Geometry: final body of the model. Coordinates: model frame, mm. A direction names the side the tool comes from. Give positions to 0.01 mm unless a question says otherwise; leave off trailing zeros. Write each loop counter-clockwise with the first axis right and the second up, starting at its lowest first coordinate (ties: lowest second). Pieces come first, ordered by that corner, then holes. Notation, with made-up numbers: M 30.25,52 L 49.25,52 A26 cw 49.25,82 Z; hole C 21,50.5 d7. An arc over 180 degrees is marked long. Use a Markdown table: item, result. Add a question column.
1) Set-up query: faces 4 (the flat face through (-103, 56, 20)), 5 (the flat face through (-201.182, 5.708, 8.948)), 6 (the flat face through (-82.379, 80.196, 19.088)), 7 (the cylindrical face through (-11.492, 18.486, 9.251)). Return all of +Z, -Z, +X, -X, +Y, -Y with unobstructed straight access to the full face (end or side cutting, diameter ignored); none if empty.
2) Section A-A on x = -62. Return the cut outline in (y, z), then the cut area to 3 significant figures.
3) Line query: line 1 (X direction, y = 16.5, z = 17); line 2 (Y direction, x = -67, z = 13). Output: solid intervals per line, ascending.
4) Pin query (flat end, axial travel): pin 1 (1.3 mm diameter, centred on x = -12.5, y = 16.5, fed in from -Z); pin 2 (5 mm diameter, centred on y = 73.5, z = 6.5, fed in from +X). Return the tip coordinate at first contact, or that it passes through.
5) Section D-D on y = 7. Return the cut outline in (x, z) (3 decimals).
6) Draft query along Y for faces 1 (the flat face through (-101, 1.85, 9)), 2 (the flat face through (-107, 96, 0)), 3 (the flat face through (-7.45, 95.64, 12.18)). Return one class per face: +Y half, -Y half, draft (parallel to the pull), parting line (faces both ways), or undercut.
7) Section B-B on y = 65. Return the cut outline in (x, z).
8) Section C-C on z = 9. Return the cut outline in (x, y), then the cut area to 3 significant figures.
```python
from build123d import *

# Parameters (mm, degrees)
PAD_DEPTH       = 20
POCKET_DEPTH    = 20
POCKET001_DEPTH = 18.15
SKETCH003_R     = 2.25
PAD001_DEPTH    = 18.05


with BuildPart() as part:
    # Sketch → Pad (new body)
    with BuildSketch(Plane.XY):
        Polygon((-8.910891, 97.1), (0, 88.189109), (0, 8.910891), (-8.910891, 0), (-198.089109, 0), (-207, 8.910891), (-207, 88.189109), (-198.089109, 97.1), align=None)
    extrude(amount=PAD_DEPTH)

    # Sketch001 (on Face10 of Pad) → Pocket (cut)
    with BuildSketch(Plane.XY.offset(20)):
        Polygon((-95.65, 66.925), (-95.65, 30.175), (-69.475, 4), (-33.025, 4), (-6.85, 30.175), (-6.85, 66.925), (-33.025, 93.1), (-69.475, 93.1), align=None)
        Polygon((-197.45, 66.925), (-197.45, 30.175), (-171.275, 4), (-134.825, 4), (-108.65, 30.175), (-108.65, 66.925), (-134.825, 93.1), (-171.275, 93.1), align=None)
    extrude(amount=-POCKET_DEPTH, mode=Mode.SUBTRACT)

    # Sketch002 (on Face4 of Pocket) → Pocket001 (cut)
    with BuildSketch(Plane(origin=(0, 0, 0), x_dir=(1, 0, 0), z_dir=(0, 0, -1))):
        Polygon((-197.323705, -1.85), (-205.15, -9.676295), (-205.15, -87.423705), (-197.323705, -95.25), (7.29, -95.25), (7.29, -1.85), align=None)
    extrude(amount=-POCKET001_DEPTH, mode=Mode.SUBTRACT)

    # Sketch003 (on Face32 of Pocket001) → Pad001 (join)
    with BuildSketch(Plane(origin=(0, 0, 18.15), x_dir=(1, 0, 0), z_dir=(0, 0, -1))):
        with Locations((-12.53, -16.49)):
            Circle(SKETCH003_R)
        with Locations((-191.771101, -16.492657)):
            Circle(SKETCH003_R)
        with Locations((-12.528899, -80.607343)):
            Circle(SKETCH003_R)
        with Locations((-191.771101, -80.607343)):
            Circle(SKETCH003_R)
    extrude(amount=PAD001_DEPTH)


solid = part.part
```
Found:
| question | item | result |
|---|---|---|
| 1 | face 4 | +Z, +X, -X, +Y, -Y |
| 1 | face 5 | -Z, +X |
| 1 | face 6 | +Z, -Z |
| 1 | face 7 | -Z |
| 2 | outline | M 0,0 L 1.85,0 L 1.85,18.15 L 4,18.15 L 4,20 L 0,20 Z; M 93.1,18.15 L 95.25,18.15 L 95.25,0 L 97.1,0 L 97.1,20 L 93.1,20 Z |
| 2 | area | 82.0 mm² |
| 3 | line 1 | -207 to -205.15, -194.02 to -189.52, -14.78 to -10.28 |
| 3 | line 2 | 0 to 1.85, 95.25 to 97.1 |
| 4 | pin 1 | z = 0.1 |
| 4 | pin 2 | x = -205.15 |
| 5 | outline | M -205.089,0 L -202.474,0 L -202.474,18.15 L -174.275,18.15 L -174.275,20 L -205.089,20 Z; M -131.825,18.15 L -72.475,18.15 L -72.475,20 L -131.825,20 Z; M -30.025,18.15 L -1.911,18.15 L -1.911,20 L -30.025,20 Z |
| 6 | face 1 | undercut |
| 6 | face 2 | draft |
| 6 | face 3 | +Y half |
| 7 | outline | M -207,0 L -205.15,0 L -205.15,18.15 L -197.45,18.15 L -197.45,20 L -207,20 Z; M -108.65,18.15 L -95.65,18.15 L -95.65,20 L -108.65,20 Z; M -6.85,18.15 L 0,18.15 L 0,20 L -6.85,20 Z |
| 8 | outline | M -207,8.91 L -198.09,0 L -8.91,0 L -7.06,1.85 L -197.32,1.85 L -205.15,9.68 L -205.15,87.42 L -197.32,95.25 L -7.06,95.25 L -8.91,97.1 L -198.09,97.1 L -207,88.19 Z; C -191.77,16.49 d4.5; C -191.77,80.61 d4.5; C -12.53,16.49 d4.5; C -12.53,80.61 d4.5 |
| 8 | area | 955 mm² |
